Part model, mm, in its own coordinate system. A direction names the side the tool comes from. Coordinates: 2 decimals unless noted, no trailing zeros. Write each loop counter-clockwise with the first axis right and the second up, starting at its lowest first coordinate (ties: lowest second). Pieces come first, ordered by that corner, then holes. Notation, with made-up numbers: M 29,31 L 44,31 A35 ccw 44,68 Z; hole C 68.5,67 d6. An arc over 180 degrees is marked long. Use a Markdown table: item, result. Add a question column.
Q1. Slice it at A-A on z = 2.25. Write the cut outline in (x, y).
Q2. Mould opens along Y. For faces 4 (the cylindrical face through (10.476, 9.632, 5.577)), 5 (the flat face through (11, 0, 11)), 6 (the flat face through (0, -15, 4)) say: released by +Y, released by -Y, zero draft, split by the parting line, or undercut.
Q3. Pin check, flat tips, straight feed: pin 1 Ø3 at (x, y) = (-12, -9) entering from +Z; pin 2 Ø5 at (y, z) = (12, 9.5) entering from +X; pin 3 Ø2 at (x, y) = (-6, 9.5) entering from +Z; pin 4 Ø2.5 at (y, z) = (4, 10) entering from -X. Stop position of each tip, or through.
Q4. Tool access for faces 1 (the flat face through (-1.2, 12, 4.9)), 2 (the flat face through (16.5, 0, 9)), 3 (the flat face through (-16.5, 0, 10)): list every direction of +Z, -Z, +X, -X, +Y, -Y with a clear straight run to the whole face (end or side of a thin tool).
Q5. Slice it at C-C on y = 9. Write the cut outline in (x, z).
Q6. Slice it at D-D on x = -7. Write the cut outline in (y, z), then the cut area to 3 significant figures.
Q7. Wall check: L1, parallel to Y at x = -12, z = 6.75; L2, parallel to X at y = -9, z = 6; L3, parallel to X at y = -10, z = 8.75. Give the ranges that are in metal, low to high. Write a range as from..to.
Q8. Slice it at B-B on x = -12. Write the cut outline in (y, z).
from build123d import *

# Parameters (mm, degrees)
F1_DEPTH = 15
F3_D     = 3.3
F4_R     = 7.7
F5_DEPTH = 12


with BuildPart() as f1:
    # F0 (on Front) → F1 (new body, symmetric)
    with BuildSketch(Plane.XZ):
        with BuildLine():
            Line((-5.4519269615, 0), (0, 0))
            Line((0, 0), (0, 5))
            ThreePointArc((0, 5), (-4.2426406871, 6.7573593129), (-6, 11))
            Line((-6, 11), (-16.5, 11))
            Line((-16.5, 11), (-16.5, 8))
            Line((-16.5, 8), (-17, 6))
            Line((-17, 6), (-17, 0))
            Line((-17, 0), (-9.5, 0))
            Line((-9.5, 0), (-5.4519269615, 0))
        make_face()
        with BuildLine():
            Line((0, 5), (0, 0))
            Line((0, 0), (5.4519269615, 0))
            Line((5.4519269615, 0), (9.5, 0))
            Line((9.5, 0), (17, 0))
            Line((17, 0), (17, 6))
            Line((17, 6), (16.5, 8))
            Line((16.5, 8), (16.5, 11))
            Line((16.5, 11), (6, 11))
            ThreePointArc((6, 11), (4.2426406871, 6.7573593129), (0, 5))
        make_face()
    extrude(amount=F1_DEPTH, both=True)

    # F3 (through all)
    with Locations(Plane(origin=(0, 0, 0), x_dir=(1, 0, 0), z_dir=(0, 0, -1))):
        with Locations((-12, 9), (-12, -9), (12, -9), (12, 9)):
            Hole(F3_D / 2)

    # F4 (on Front) → F5 (cut, symmetric)
    with BuildSketch(Plane.XZ):
        with Locations((0, 11)):
            Circle(F4_R)
    extrude(amount=F5_DEPTH, both=True, mode=Mode.SUBTRACT)


solid = f1.part
Recorded:
| question | item | result |
|---|---|---|
| 1 | outline | M -17,-15 L 17,-15 L 17,15 L -17,15 Z; hole C -12,-9 d3.3; hole C -12,9 d3.3; hole C 12,-9 d3.3; hole C 12,9 d3.3 |
| 2 | face 4 | undercut |
| 2 | face 5 | zero draft |
| 2 | face 6 | released by -Y |
| 3 | pin 1 | through |
| 3 | pin 2 | x = 16.75 |
| 3 | pin 3 | z = 7.79 |
| 3 | pin 4 | x = -16.5 |
| 4 | face 1 | +Z |
| 4 | face 2 | +Z, +X, +Y, -Y |
| 4 | face 3 | +Z, -X, +Y, -Y |
| 5 | outline | M -17,0 L -13.65,0 L -13.65,11 L -16.5,11 L -16.5,8 L -17,6 Z; M -10.35,0 L 10.35,0 L 10.35,11 L 7.7,11 A7.7 cw -7.7,11 L -10.35,11 Z; M 13.65,0 L 17,0 L 17,6 L 16.5,8 L 16.5,11 L 13.65,11 Z |
| 6 | outline | M -15,0 L 15,0 L 15,11 L 12,11 L 12,7.79 L -12,7.79 L -12,11 L -15,11 Z |
| 6 | area | 253 mm² |
| 7 | L1 | -15..-10.65, -7.35..7.35, 10.65..15 |
| 7 | L2 | -17..-13.65, -10.35..-5.86, 5.86..10.35, 13.65..17 |
| 7 | L3 | -16.5..-13.31, -10.69..-7.36, 7.36..10.69, 13.31..16.5 |
| 8 | outline | M -15,0 L -10.65,0 L -10.65,11 L -15,11 Z; M -7.35,0 L 7.35,0 L 7.35,11 L -7.35,11 Z; M 10.65,0 L 15,0 L 15,11 L 10.65,11 Z |
